The listing builds one solid part. Answer for the finished solid, in the listing's coordinates (mm). A direction names the side the tool comes from. Round coordinates to 2 decimals unless told otherwise and drop trailing zeros. Loops run counter-clockwise (first coordinate to the right, second up) from the corner with the lowest first, then second, coordinate; pieces in that order, holes last. Notation, with made-up numbers: (-6, 50) -> (12, 50) arc R38 cw to (12, 88) -> close; hole circle Ø6 at (-31, 31.5). An arc over 180 degrees is marked (long way). One line per question, with ' | ' between items.
from build123d import *

# Parameters (mm, degrees)
BOSS_EXTRUDE1_DEPTH      = 800
SKETCH2_W                = 300
SKETCH2_H                = 200
CUT_EXTRUDE1_DEPTH       = 125
BOSS_EXTRUDE2_DEPTH      = 100
BOSS_EXTRUDE2_DEPTH_BACK = 100
SKETCH4_R                = 12.5
SKETCH5_W                = 1800
SKETCH5_H                = 700
CUT_EXTRUDE2_DEPTH       = 75
BOSS_EXTRUDE3_DEPTH      = 900
BOSS_EXTRUDE3_DEPTH_BACK = 900
SKETCH8_W                = 50
SKETCH8_H                = 75
BOSS_EXTRUDE4_DEPTH      = 120
BOSS_EXTRUDE5_DEPTH      = 120
CUT_EXTRUDE4_DEPTH       = 740
CUT_EXTRUDE4_DEPTH_BACK  = 40
SKETCH7_R                = 7.5
BOSS_EXTRUDE6_DEPTH      = 25
BOSS_EXTRUDE6_DEPTH_BACK = 25
SKETCH12_R               = 9.525
SKETCH13_W               = 31.75
SKETCH13_H               = 68.5
CUT_EXTRUDE5_DEPTH       = 1381.258967746


with BuildPart() as part:
    # Sketch1 → Boss-Extrude1 (new body)
    with BuildSketch(Plane.XY):
        Polygon((-900, 182.495667244), (900, 182.495667244), (900, -67.504332756), (500, -67.504332756), (500, -267.504332756), (-500, -267.504332756), (-500, -67.504332756), (-900, -67.504332756), align=None)
    extrude(amount=BOSS_EXTRUDE1_DEPTH)

    # Sketch2 → Cut-Extrude1 (cut)
    with BuildSketch(Plane.XZ.offset(67.504332756)):
        with Locations((700, 125)):
            Rectangle(SKETCH2_W, SKETCH2_H)
        with Locations((-700, 125)):
            Rectangle(SKETCH2_W, SKETCH2_H)
        with Locations((-700, 675)):
            Rectangle(SKETCH2_W, SKETCH2_H)
        with Locations((700, 675)):
            Rectangle(SKETCH2_W, SKETCH2_H)
    extrude(amount=-CUT_EXTRUDE1_DEPTH, mode=Mode.SUBTRACT)

    # Sketch4 → Boss-Extrude2 (add, two sides: drawn at the far end of the back side and taken through both)
    # profile 1 of 2: a face of its own
    with BuildSketch(Plane(origin=(0, 0, 400), x_dir=(-1, 0, 0), z_dir=(0, 0, -1)).offset(-BOSS_EXTRUDE2_DEPTH_BACK)):
        with BuildLine():
            Line((-775, -67.504332756), (-625, -67.504332756))
            ThreePointArc((-625, -67.504332756), (-700, -142.504332756), (-775, -67.504332756))
        make_face()
        with Locations((-700, -117.504332756)):
            Circle(SKETCH4_R, mode=Mode.SUBTRACT)
    # profile 2 of 2: a face of its own
    with BuildSketch(Plane(origin=(0, 0, 400), x_dir=(-1, 0, 0), z_dir=(0, 0, -1)).offset(-BOSS_EXTRUDE2_DEPTH_BACK)):
        with BuildLine():
            Line((625, -67.504332756), (775, -67.504332756))
            ThreePointArc((775, -67.504332756), (700, -142.504332756), (625, -67.504332756))
        make_face()
        with Locations(Location((700, -117.504332756, 0), (0, 0, 180))):
            Circle(SKETCH4_R, mode=Mode.SUBTRACT)
    extrude(amount=BOSS_EXTRUDE2_DEPTH + BOSS_EXTRUDE2_DEPTH_BACK)

    # Sketch5 → Cut-Extrude2 (cut)
    with BuildSketch(Plane(origin=(0, 182.495667244, 0), x_dir=(1, 0, 0), z_dir=(0, 1, 0))):
        with Locations((0, -400)):
            Rectangle(SKETCH5_W, SKETCH5_H)
    extrude(amount=-CUT_EXTRUDE2_DEPTH, mode=Mode.SUBTRACT)

    # Sketch8 → Boss-Extrude3 (add, two sides: drawn at the far end of the back side and taken through both)
    with BuildSketch(Plane(origin=(0, 0, 0), x_dir=(0, 0, -1), z_dir=(1, 0, 0)).offset(-BOSS_EXTRUDE3_DEPTH_BACK)):
        with Locations((-715, 144.995667244)):
            Rectangle(SKETCH8_W, SKETCH8_H)
        with Locations((-85, 144.995667244)):
            Rectangle(SKETCH8_W, SKETCH8_H)
    extrude(amount=BOSS_EXTRUDE3_DEPTH + BOSS_EXTRUDE3_DEPTH_BACK)

    # Sketch9 → Boss-Extrude4 (add)
    with BuildSketch(Plane(origin=(900, 0, 0), x_dir=(0, 0, -1), z_dir=(1, 0, 0))):
        Polygon((-800, 182.495667244), (-750, 182.495667244), (-750, 107.495667244), (-740, 107.495667244), (-740, 182.495667244), (-690, 182.495667244), (-690, 107.495667244), (-110, 107.495667244), (-110, 182.495667244), (-60, 182.495667244), (-60, 107.495667244), (-50, 107.495667244), (-50, 182.495667244), (0, 182.495667244), (0, -67.504332756), (-800, -67.504332756), align=None)
    extrude(amount=BOSS_EXTRUDE4_DEPTH)

    # Sketch10 → Boss-Extrude5 (add)
    with BuildSketch(Plane.ZY.offset(900)):
        Polygon((800, 182.495667244), (750, 182.495667244), (750, 107.495667244), (740, 107.495667244), (740, 182.495667244), (690, 182.495667244), (690, 107.495667244), (110, 107.495667244), (110, 182.495667244), (60, 182.495667244), (60, 107.495667244), (50, 107.495667244), (50, 182.495667244), (0, 182.495667244), (0, -67.504332756), (800, -67.504332756), align=None)
    extrude(amount=BOSS_EXTRUDE5_DEPTH)

    # Sketch7 → Cut-Extrude4 (cut, two sides: drawn at the far end of the back side and taken through both)
    with BuildSketch(Plane(origin=(0, 0, 750), x_dir=(-1, 0, 0), z_dir=(0, 0, -1)).offset(-CUT_EXTRUDE4_DEPTH_BACK)):
        with Locations(Location((-35, 144.995667244, 0), (0, 0, 180))):
            Circle(SKETCH7_R)
        with Locations(Location((-350, 144.995667244, 0), (0, 0, 180))):
            Circle(SKETCH7_R)
        with Locations(Location((-310, 144.995667244, 0), (0, 0, 180))):
            Circle(SKETCH7_R)
        with Locations(Location((10, 144.995667244, 0), (0, 0, 180))):
            Circle(SKETCH7_R)
        with BuildLine():
            Line((960, 137.495667244), (510, 137.495667244))
            ThreePointArc((510, 137.495667244), (502.5, 144.995667244), (510, 152.495667244))
            Line((510, 152.495667244), (960, 152.495667244))
            ThreePointArc((960, 152.495667244), (967.5, 144.995667244), (960, 137.495667244))
        make_face()
        with BuildLine():
            Line((-1000, 152.495667244), (-675, 152.495667244))
            ThreePointArc((-675, 152.495667244), (-667.5, 144.995667244), (-675, 137.495667244))
            Line((-675, 137.495667244), (-1000, 137.495667244))
            ThreePointArc((-1000, 137.495667244), (-1007.5, 144.995667244), (-1000, 152.495667244))
        make_face()
    extrude(amount=CUT_EXTRUDE4_DEPTH + CUT_EXTRUDE4_DEPTH_BACK, mode=Mode.SUBTRACT)

    # Sketch12 → Boss-Extrude6 (add, two sides: drawn at the far end of the back side and taken through both)
    # profile 1 of 2: a face of its own
    with BuildSketch(Plane(origin=(0, 0, 400), x_dir=(-1, 0, 0), z_dir=(0, 0, -1)).offset(-BOSS_EXTRUDE6_DEPTH_BACK)):
        with BuildLine():
            Line((72.5, 107.495667244), (72.5, 163.595667244))
            ThreePointArc((72.5, 163.595667244), (68.868124087, 172.363791331), (60.1, 175.995667244))
            Line((60.1, 175.995667244), (59.9, 175.995667244))
            ThreePointArc((59.9, 175.995667244), (51.131875913, 172.363791331), (47.5, 163.595667244))
            Line((47.5, 163.595667244), (47.5, 107.495667244))
            Line((47.5, 107.495667244), (72.5, 107.495667244))
        make_face()
        with Locations((60, 160.995667244)):
            Circle(SKETCH12_R, mode=Mode.SUBTRACT)
    # profile 2 of 2: a face of its own
    with BuildSketch(Plane(origin=(0, 0, 400), x_dir=(-1, 0, 0), z_dir=(0, 0, -1)).offset(-BOSS_EXTRUDE6_DEPTH_BACK)):
        with BuildLine():
            Line((-345, 107.495667244), (-345, 163.595667244))
            ThreePointArc((-345, 163.595667244), (-348.631875913, 172.363791331), (-357.4, 175.995667244))
            Line((-357.4, 175.995667244), (-357.6, 175.995667244))
            ThreePointArc((-357.6, 175.995667244), (-366.368124087, 172.363791331), (-370, 163.595667244))
            Line((-370, 163.595667244), (-370, 107.495667244))
            Line((-370, 107.495667244), (-345, 107.495667244))
        make_face()
        with Locations((-357.5, 160.995667244)):
            Circle(SKETCH12_R, mode=Mode.SUBTRACT)
    extrude(amount=BOSS_EXTRUDE6_DEPTH + BOSS_EXTRUDE6_DEPTH_BACK)

    # Sketch13 → Cut-Extrude5 (cut, through all)
    with BuildSketch(Plane.ZY.offset(72.5)):
        with Locations((400, 141.745667244)):
            Rectangle(SKETCH13_W, SKETCH13_H)
    extrude(amount=-CUT_EXTRUDE5_DEPTH, mode=Mode.SUBTRACT)


solid = part.part
Q1. A cutting plane is placed at B-B on x = -232. Give the vertices of the cut face in (y, z).
Numbers:
outline: (-267.5, 0) -> (182.5, 0) -> (182.5, 50) -> (107.5, 50) -> (107.5, 60) -> (182.5, 60) -> (182.5, 110) -> (107.5, 110) -> (107.5, 690) -> (182.5, 690) -> (182.5, 740) -> (107.5, 740) -> (107.5, 750) -> (182.5, 750) -> (182.5, 800) -> (-267.5, 800) -> close
Q2. For faces 1 (the face through (698, -6, 775)), 2 (the face through (14, 146, 60)), 3 (the face through (-701, -96, 300)), determine the directions among +Z, -Z, +X, -X, +Y, -Y from which every point of the face is accessible in a straight line to the end or side of a thin tool.
Numbers:
face 1: -Y | face 2: +X, -X, +Y | face 3: -Z, -X, -Y
Q3. A cutting plane is placed at C-C on z = 87.5. Give the vertices of the cut face in (x, y), plus the area to 3 significant figures.
Numbers:
outline: (-1020, -67.5) -> (-850, -67.5) -> (-850, 57.5) -> (-550, 57.5) -> (-550, -67.5) -> (-500, -67.5) -> (-500, -267.5) -> (500, -267.5) -> (500, -67.5) -> (550, -67.5) -> (550, 57.5) -> (850, 57.5) -> (850, -67.5) -> (1020, -67.5) -> (1020, 182.5) -> (-1020, 182.5) -> close; hole (-960, 137.5) -> (-510, 137.5) arc R7.5 ccw to (-510, 152.5) -> (-960, 152.5) arc R7.5 ccw to start; hole circle Ø15 at (-10, 145); hole circle Ø15 at (35, 145); hole circle Ø15 at (310, 145); hole circle Ø15 at (350, 145); hole (675, 137.5) -> (1000, 137.5) arc R7.5 ccw to (1000, 152.5) -> (675, 152.5) arc R7.5 ccw to start | area: 622,000 mm^2
Q4. Find the intervals of material crossed by line 1 (X direction, y = 22, z = 587); line 2 (Z direction, x = 154.5, y = 163); line 3 (Y direction, x = -60, z = 419), in increasing order. Write a range as from..to.
Numbers:
line 1: -1020..-850, -550..550, 850..1020 | line 2: 0..50, 60..110, 690..740, 750..800 | line 3: -267.5..151.47, 170.52..176
Q5. A cutting plane is placed at A-A on z = 275. Give the vertices of the cut face in (x, y), plus the area to 3 significant figures.
Numbers:
outline: (-1020, -67.5) -> (-500, -67.5) -> (-500, -267.5) -> (500, -267.5) -> (500, -67.5) -> (1020, -67.5) -> (1020, 107.5) -> (-1020, 107.5) -> close | area: 557,000 mm^2
Q6. Given pin 1 Ø12 at (y, z) = (-178, 149) entering from -X; pin 2 Ø8 at (y, z) = (-72.5, 366.5) entering from -X; pin 3 Ø12 at (x, z) = (735, 402) entering from -Y, each flat-ended and moving along its own axis, determine where each tip first touches the part or whether it passes through.
Numbers:
pin 1: x = -500 | pin 2: x = -774.99 | pin 3: y = -136.67
Q7. For a pull along Y with two mould halves and no side action, classify faces 4 (the face through (699, -96, 500)), 5 (the face through (840, 152.496, 85)), 6 (the face through (698.351, -142.486, 401.4)) as pulls with the +Y half, pulls with the -Y half, needs draft (parallel to the pull), parting line crosses it, or undercut.
Numbers:
face 4: needs draft | face 5: undercut | face 6: pulls with the -Y half
